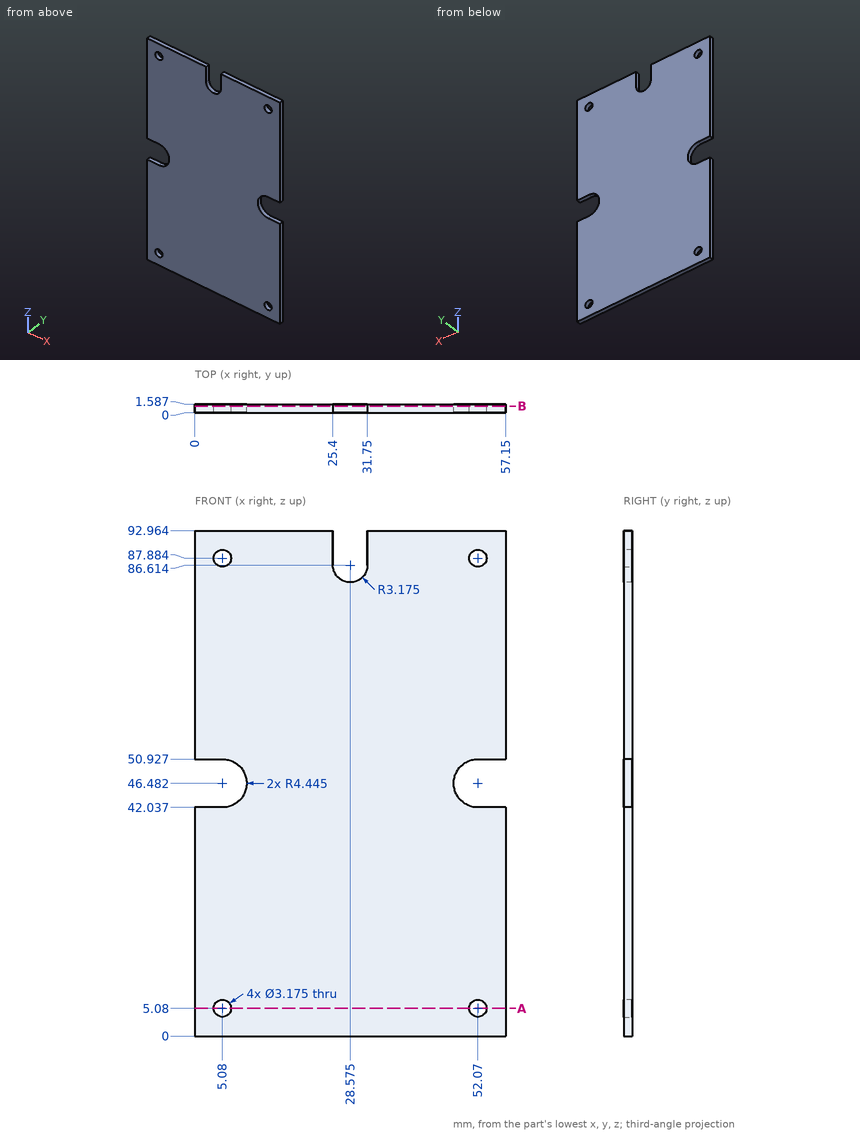
Can you work these out from the drawing? Everything is in mm from the part's minimum corner. Give positions to 0.01 mm unless a question says otherwise; leave off trailing zeros. Loops run counter-clockwise (first coordinate to the right, second up) from the corner with the lowest first, then second, coordinate; pieces in that order, holes last. Notation, with made-up numbers: (29.5, 23) -> (84.5, 23) arc R20 cw to (84.5, 60) -> close; hole circle Ø2 at (-9.75, 78). An arc over 180 degrees is marked (long way). Return JSON: item names as keys, results as strings.
Q1. I want a section at B-B, the plane y = 1.2. Count the separate pieces of the cut face and the enclosed holes in it, then the cut area to 3 significant figures.
Checks:
{"separate pieces": "1", "enclosed holes": "4", "area": "5,070 mm2"}
Q2. I want a section at A-A, the plane z = 5.08. List the corners of the cut face in (x, y) for me.
Checks:
{"outline": "(0, 0) -> (3.49, 0) -> (3.49, 1.59) -> (0, 1.59) -> close; (6.67, 0) -> (50.48, 0) -> (50.48, 1.59) -> (6.67, 1.59) -> close; (53.66, 0) -> (57.15, 0) -> (57.15, 1.59) -> (53.66, 1.59) -> close"}
Q3. For pin 1 Ø2.5 at (x, z) = (52.07, 87.884) entering from -Y, with a flat end and sliding along its axis, tell me the tip position at first contact or that it passes through.
Checks:
{"pin 1": "passes through"}
Q4. I need wall thicknesses on probe 1 along X at (y, z) = (1, 5.08); probe 2 along Z at (x, y) = (54, 0.1) (1 decimal); probe 3 along Z at (x, y) = (30.5, 0.65). Which ranges of each line are inside material? Lowest first, please.
Checks:
{"probe 1": "x = 0 to 3.49, 6.67 to 50.48, 53.66 to 57.15", "probe 2": "z = 0 to 42, 50.9 to 93", "probe 3": "z = 0 to 84.09"}
